Autodesk Inventor part; units mm, degrees
ref_plane "YZ Plane" through (0, 0, 0) normal (1, 0, 0) x (0, 1, 0)
ref_plane "XZ Plane" through (0, 0, 0) normal (0, 1, 0) x (-1, 0, 0)
ref_plane "XY Plane" through (0, 0, 0) normal (0, 0, 1) x (1, 0, 0)
sketch "Sketch1" plane through (0, 0, 0) normal (0, 0, 1) x (1, 0, 0)
  circle A0 centre (0, 0) radius 2.5
  dimension "d0" = 5
extrude "Extrusion1" add sketch "Sketch1" along normal blind 30
sketch "Sketch2" plane through (0, 0, 30) normal (0, 0, 1) x (1, 0, 0)
  circle A0 centre (0, 0) radius 2.5
  circle A1 centre (0, 0) radius 1.5
  dimension "d3" = 3
extrude "Extrusion2" add sketch "Sketch2" along normal blind 3 contours A1
thread "Thread1"
sketch "Sketch3" plane through (0, 0, 0) normal (0, 0, -1) x (-1, 0, 0)
  circle A0 centre (0, 0) radius 2.5
  circle A1 centre (0, 0) radius 1.5
  dimension "d8" = 3
extrude "Extrusion3" add sketch "Sketch3" along normal blind 3 contours A1
thread "Thread2"
properties part number "spacer 5cm"
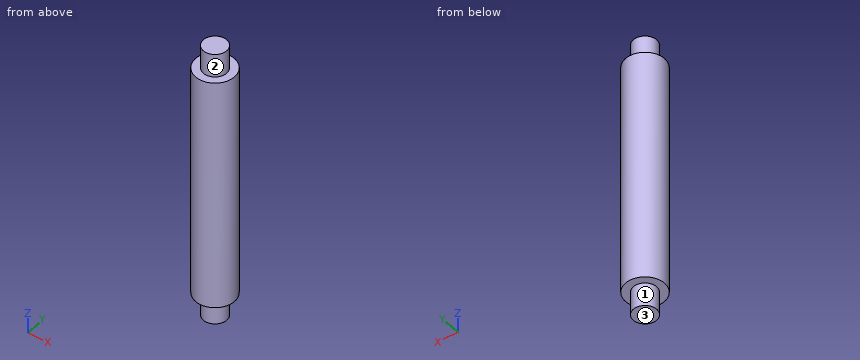
Can you work these out from the model? Positions are in its coordinate system, mm. Face numbers are marked on the shaded views. A direction names the side the tool comes from. Give positions to 0.01 mm unless a question says otherwise; leave off trailing zeros. Loops run counter-clockwise (first coordinate to the right, second up) from the corner with the lowest first, then second, coordinate; pieces in that order, holes last. Notation, with made-up numbers: M 88.5,0.5 L 139.5,0.5 A31 ccw 139.5,30.5 Z; hole C -25,7 d3. An arc over 180 degrees is marked long. One line per item, written item: value. Start each with the question number.
1) If I drill on line 1 (Y direction, x = 2, z = 12); line 2 (X direction, y = -0.15, z = 23); line 3 (Z direction, x = 2.15, y = 0.7), over which ranges is the centre line in solid material (lowest first)? Write a range as [from, to].
2) If we section it at D-D, the plane y = 2.1: Write out the boundary of the cut face in (x, z), and give its area (3 significant figures).
3) If we section it at A-A, the plane x = 0: Write out the boundary of the cut face in (y, z).
4) If we section it at C-C, the plane z = 13.5: Write out the boundary of the cut face in (x, y).
5) On a 3-axis mill with a long thin cutter (end or side, diameter ignored), from which of +Z, -Z, +X, -X, +Y, -Y can I reach the whole of each face in a straight line? I mean the marked faces 1, 2 and 3. Say none if no direction works.
Completed:
1. line 1: y = [-1.5, 1.5]
1. line 2: x = [-2.5, 2.5]
1. line 3: z = [0, 30]
2. outline: M -1.36,0 L 1.36,0 L 1.36,30 L -1.36,30 Z
2. area: 81.4 mm^2
3. outline: M -2.5,0 L -1.5,0 L -1.5,-3 L 1.5,-3 L 1.5,0 L 2.5,0 L 2.5,30 L 1.5,30 L 1.5,33 L -1.5,33 L -1.5,30 L -2.5,30 Z
4. outline: C 0,0 d5
5. face 1: -Z
5. face 2: +Z
5. face 3: -Z, +X, -X, +Y, -Y
